Geometry: final body of the model. Coordinates: model frame, mm. A direction names the side the tool comes from. Give positions to 0.01 mm unless a question says otherwise; leave off trailing zeros. Order: outer loops, then holes, each group sorted by start corner. A loop starts at its lowest first (then second) coordinate and runs counter-clockwise, first axis right, second up. Notation, with made-up numbers: M 33.5,36.5 L 90.5,36.5 A12 ccw 90.5,43.5 Z; hole C 14,2.25 d6. An arc over 180 degrees is marked long. Use CSV: the item, a comma, the result in double quotes.
```python
from build123d import *

# Parameters (mm, degrees)
BOSS_EXTRU_1_DEPTH      = 3.5
ESQUISSE3_R             = 1
ENL_V_MAT_EXTRU_1_DEPTH = 4
ESQUISSE4_R             = 1
ENL_V_MAT_EXTRU_2_DEPTH = 10
ENL_V_MAT_EXTRU_3_DEPTH = 57.011159602
CONG_1_SIZE             = 5
CONG_1_SIZE_2           = 3
ENL_V_MAT_EXTRU_7_DEPTH = 6
CONG_4_R                = 2
CONG_5_R                = 2


with BuildPart() as part:
    # Esquisse1 → Boss.-Extru.1 (new body)
    with BuildSketch(Plane.XY):
        with BuildLine():
            Line((0, 0), (10, 0))
            Line((10, 0), (10, -52.5))
            ThreePointArc((10, -52.5), (7.5, -55), (5, -52.5))
            Line((5, -52.5), (5, -5))
            Line((5, -5), (0, -5))
            Line((0, -5), (0, 0))
        make_face()
    extrude(amount=BOSS_EXTRU_1_DEPTH)

    # Esquisse3 → Enlèv. mat.-Extru.1 (cut)
    with BuildSketch(Plane(origin=(0, 0, 0), x_dir=(-1, 0, 0), z_dir=(0, 0, -1))):
        with Locations((-7.5, -52.5)):
            Circle(ESQUISSE3_R)
    extrude(amount=-ENL_V_MAT_EXTRU_1_DEPTH, mode=Mode.SUBTRACT)

    # Esquisse4 → Enlèv. mat.-Extru.2 (cut)
    with BuildSketch(Plane.XY.offset(3.5)):
        with Locations((7.5, -36.5)):
            Circle(ESQUISSE4_R)
    extrude(amount=-ENL_V_MAT_EXTRU_2_DEPTH, mode=Mode.SUBTRACT)

    # Esquisse5 → Enlèv. mat.-Extru.3 (cut, through all)
    with BuildSketch(Plane.XY.offset(3.5)):
        Polygon((0, 0), (1.700931961, 0), (0, -5), align=None)
    extrude(amount=-ENL_V_MAT_EXTRU_3_DEPTH, mode=Mode.SUBTRACT)

    # Congé1
    # a fillet whose section is not a circle: 5, 3 mm, written as the material it adds along each edge
    with BuildSketch(Plane(origin=(5, -5, 0), x_dir=(-1, 0, 0), z_dir=(0, 0, 1))) as cong_1_piece_1_section:
        with BuildLine():
            Bezier((CONG_1_SIZE, 0), (0, 0), (0, CONG_1_SIZE_2), weights=[1, 1.5, 1])
            Line((0, CONG_1_SIZE_2), (0, 0))
            Line((0, 0), (CONG_1_SIZE, 0))
        make_face()
    cong_1_piece_1 = extrude(amount=3.5, mode=Mode.PRIVATE)
    cong_1_piece_1 = split(cong_1_piece_1, bisect_by=Plane(origin=(0.518616131, -3.47549419, 0), z_dir=(0.9467189518296611, -0.32206090456084224, 0)), keep=Keep.TOP, mode=Mode.PRIVATE)
    add(cong_1_piece_1)

    # Esquisse11 → Enlèv. mat.-Extru.7 (cut)
    with BuildSketch(Plane.XY.offset(3.5)):
        with BuildLine():
            Line((5.143373152, -7.30566223), (4.982244072, -8.50993083))
            Line((4.982244072, -8.50993083), (2.030783729, -5.080870965))
            add(Edge.make_bspline(
                [(2.030783729, -5.080870965), (4.543708127, -5.064842627), (5.143373152, -7.30566223)],
                knots=[0, 0, 0, 1, 1, 1], degree=2))
        make_face()
    extrude(amount=-ENL_V_MAT_EXTRU_7_DEPTH, mode=Mode.SUBTRACT)

    # Congé4
    cong_4_edges = [part.edges().sort_by_distance(p)[0] for p in [
        (5, -8.377224145, 1.75),
        (5.143373152, -7.30566223, 1.75),
    ]]
    fillet(cong_4_edges, radius=CONG_4_R)

    # Congé5
    cong_5_edges = [part.edges().sort_by_distance(p)[0] for p in [
        (2.032105754, -5.080862688, 1.75),
    ]]
    fillet(cong_5_edges, radius=CONG_5_R)


solid = part.part
```
1. Line query: line 1 (Y direction, x = 7.5, z = 2.4); line 2 (Y direction, x = 7, z = 0.9); line 3 (X direction, y = -38, z = 3.05). Output: solid intervals per line, ascending.
Answer:
line 1,"-55 to -53.5, -51.5 to -37.5, -35.5 to 0"
line 2,"-54.95 to -53.37, -51.63 to -37.37, -35.63 to 0"
line 3,"5 to 10"
2. Reachability of faces 1 (the face through (5, -31, 2)), 2 (the face through (7, -22, 0)) from +Z, -Z, +X, -X, +Y, -Y: full face, straight path, thin tool, end or side. Return the list, or none.
Answer:
face 1,"+Z, -Z, -X, -Y"
face 2,"-Z, +X, -X, +Y, -Y"
3. Section D-D, the plane y = -16.5. Return the cut outline in (x, z), plus the area to 3 significant figures.
Answer:
outline,"M 5,0 L 10,0 L 10,3.5 L 5,3.5 Z"
area,"17.5 mm2"
4. Pin query (flat end, axial travel): pin 1 Ø1 at (y, z) = (-40, 1.5) entering from -X. Return the tip coordinate at first contact, or that it passes through.
Answer:
pin 1,"x = 5"
5. Section C-C, the plane z = 1.6. Give the number of separate pieces and of enclosed holes in the cut face, plus the area to 3 significant figures.
Answer:
separate pieces,"1"
enclosed holes,"2"
area,"288 mm2"
6. Section B-B, the plane x = 7.5. Return the cut outline in (y, z).
Answer:
outline,"M -55,0 L -53.5,0 L -53.5,3.5 L -55,3.5 Z; M -51.5,0 L -37.5,0 L -37.5,3.5 L -51.5,3.5 Z; M -35.5,0 L 0,0 L 0,3.5 L -35.5,3.5 Z"
7. Pull-direction query (X, two-part tool) for faces 3 (the face through (7, -22, 3.5)), 4 (the face through (7.37, -35.51, 1.77)), 5 (the face through (0.86, -2.47, 1.77)), 6 (the face through (7.6, -55, 1.7)); classes: +X half, -X half, draft (parallel to the pull), parting line (faces both ways), or undercut.
Answer:
face 3,"draft"
face 4,"undercut"
face 5,"-X half"
face 6,"parting line"
8. Section A-A, the plane y = -36.5. Return the cut outline in (x, z).
Answer:
outline,"M 5,0 L 6.5,0 L 6.5,3.5 L 5,3.5 Z; M 8.5,0 L 10,0 L 10,3.5 L 8.5,3.5 Z"
